Design review of the part built by this model. Coordinates are the model's own, in mm. Coordinates: 2 decimals unless noted, no trailing zeros. Write each loop counter-clockwise with the first axis right and the second up, starting at its lowest first coordinate (ties: lowest second). Pieces come first, ordered by that corner, then holes. Notation, with made-up numbers: (-30, 58.5) -> (14, 58.5) arc R12 cw to (14, 70.5) -> close; hole circle Ø1 at (12.5, 3). An arc over 180 degrees is marked (long way). One line per question, with ' | ' between items. Start each with the question number.
Q1. Add section D-D on x = 14. State the section outline as (y, z) points, and give its area (3 significant figures).
Q2. Wall thickness on probe 1 along X at (y, z) = (0, 30) (3 decimals); probe 2 along X at (y, z) = (6.5, 33.5): over which ranges is each line inside the solid? List them lowest first.
Q3. Add section C-C on x = 7. State the section outline as (y, z) points.
Q4. Add section B-B on y = 0. State the section outline as (x, z) points (1 decimal).
Q5. For P1, Ø2, axis at y = 2, z = 19, coming from the -X side; P2, Ø10, axis at x = -12.5, z = 21, coming from the +Y side; P3, Ø6, axis at x = 9.5, z = 35, coming from the +Y side, all flat-tipped, find the tip position at first contact; note any pin that passes through.
Q6. Draft analysis for pull direction Y (two halves, no side actions). For faces 1 (the flat face through (2, 12, 39.649)), 2 (the cylindrical face through (14.664, 6.08, 23.953)), 3 (the cylindrical face through (-11.99, -0.53, 27.63)), state which applies: pulls with the +Y half, pulls with the -Y half, needs draft (parallel to the pull), parting line crosses it, or undercut.
Q7. Add section A-A on x = 0. State the section outline as (y, z) points (1 decimal).
Autodesk Inventor part; units mm, degrees
ref_plane "YZ Plane" through (0, 0, 0) normal (1, 0, 0) x (0, 1, 0)
ref_plane "XZ Plane" through (0, 0, 0) normal (0, 1, 0) x (-1, 0, 0)
ref_plane "XY Plane" through (0, 0, 0) normal (0, 0, 1) x (1, 0, 0)
sketch "Sketch1" plane through (0, 0, 0) normal (0, 0, 1) x (1, 0, 0)
  circle A0 centre (0, 0) radius 15.875
  circle A1 centre (0, 0) radius 12
  dimension "d0" = 31.75
  dimension "d1" = 24
extrude "Extrusion1" add sketch "Sketch1" along normal blind 39.6494
sketch "Sketch2" plane through (0, 0, 0) normal (1, 0, 0) x (0, 1, 0)
  circle A0 centre (0, 0) radius 15.1765
  dimension "d4" = 30.353
extrude "Extrusion2" cut sketch "Sketch2" along normal through all both and the other way through all
properties part number "DPLX_P019_Camera Shroud_RevA" material "Aluminum 6061"
Output values:
1) outline: (-7.48, 13.2) arc R15.18 cw to (7.48, 13.2) -> (7.48, 39.65) -> (-7.48, 39.65) -> close | area: 376 mm2
2) probe 1: x = -15.875 to -12, 12 to 15.875 | probe 2: x = -14.48 to -10.09, 10.09 to 14.48
3) outline: (-14.25, 5.23) arc R15.18 cw to (-9.75, 11.63) -> (-9.75, 39.65) -> (-14.25, 39.65) -> close; (9.75, 11.63) arc R15.18 cw to (14.25, 5.23) -> (14.25, 39.65) -> (9.75, 39.65) -> close
4) outline: (-15.9, 15.2) -> (-12, 15.2) -> (-12, 39.6) -> (-15.9, 39.6) -> close; (12, 15.2) -> (15.9, 15.2) -> (15.9, 39.6) -> (12, 39.6) -> close
5) P1: stops at x = -15.84 | P2: stops at y = 13.99 | P3: stops at y = 14.48
6) face 1: needs draft | face 2: parting line crosses it | face 3: undercut
7) outline: (-15.9, 0) -> (-15.2, 0) arc R15.2 cw to (-12, 9.3) -> (-12, 39.6) -> (-15.9, 39.6) -> close; (12, 9.3) arc R15.2 cw to (15.2, 0) -> (15.9, 0) -> (15.9, 39.6) -> (12, 39.6) -> close
